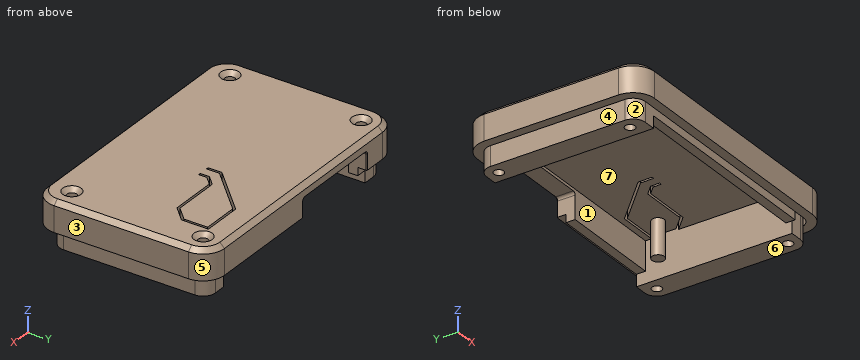
```python
from build123d import *

# Parameters (mm, degrees)
PAD002_DEPTH    = 9.9
POCKET004_DEPTH = 10
PAD003_DEPTH    = 16.4
SKETCH011_W     = 67.75
SKETCH011_H     = 3
PAD004_DEPTH    = 12.5
POCKET005_DEPTH = 13
SKETCH010_R     = 1.6
POCKET006_DEPTH = 19.401
SKETCH012_R     = 2
PAD005_DEPTH    = 14.6
POCKET007_DEPTH = 3
CHAMFER_SIZE    = 1.5
CHAMFER002_SIZE = 1.4
CHAMFER004_SIZE = 0.25


with BuildPart() as part:
    # Sketch006 → Pad002 (new body)
    with BuildSketch(Plane.XY.offset(18)):
        with BuildLine():
            ThreePointArc((-18.5, 103), (-23.449747, 100.949747), (-25.5, 96))
            Line((-25.5, 52), (-25.5, 96))
            ThreePointArc((-25.5, 52), (-23.449747, 47.050253), (-18.5, 45))
            Line((57.25, 45), (-18.5, 45))
            ThreePointArc((57.25, 45), (62.199747, 47.050253), (64.25, 52))
            Line((64.25, 96), (64.25, 52))
            ThreePointArc((64.25, 96), (62.199747, 100.949747), (57.25, 103))
            Line((-18.5, 103), (57.25, 103))
        make_face()
    extrude(amount=-PAD002_DEPTH)

    # Sketch007 → Pocket004 (cut)
    with BuildSketch(Plane.XY.offset(15)):
        with BuildLine():
            ThreePointArc((-18.5, 100), (-21.328427, 98.828427), (-22.5, 96))
            Line((-22.5, 52), (-22.5, 96))
            ThreePointArc((-22.5, 52), (-21.328427, 49.171573), (-18.5, 48))
            Line((57.25, 48), (-18.5, 48))
            ThreePointArc((57.25, 48), (60.078427, 49.171573), (61.25, 52))
            Line((61.25, 96), (61.25, 52))
            ThreePointArc((61.25, 96), (60.078427, 98.828427), (57.25, 100))
            Line((-18.5, 100), (57.25, 100))
        make_face()
    extrude(amount=-POCKET004_DEPTH, mode=Mode.SUBTRACT)

    # Sketch008 → Pad003 (join)
    with BuildSketch(Plane.XY.offset(18)):
        with BuildLine():
            ThreePointArc((-22.5, 52), (-21.328427, 49.171573), (-18.5, 48))
            Line((-14.5, 48), (-18.5, 48))
            Line((-14.5, 100), (-14.5, 48))
            Line((-18.5, 100), (-14.5, 100))
            ThreePointArc((-18.5, 100), (-21.328427, 98.828427), (-22.5, 96))
            Line((-22.5, 52), (-22.5, 96))
        make_face()
        with BuildLine():
            ThreePointArc((61.25, 96), (60.078427, 98.828427), (57.25, 100))
            Line((53.25, 100), (57.25, 100))
            Line((53.25, 49), (53.25, 100))
            Line((57.25, 49), (53.25, 49))
            ThreePointArc((57.25, 49), (60.078427, 50.171573), (61.25, 53))
            Line((61.25, 96), (61.25, 53))
        make_face()
    extrude(amount=-PAD003_DEPTH)

    # Sketch011 → Pad004 (join)
    with BuildSketch(Plane.XY.offset(18)):
        with Locations((19.375, 98.5)):
            Rectangle(SKETCH011_W, SKETCH011_H)
        with Locations((19.375, 49.5)):
            Rectangle(SKETCH011_W, SKETCH011_H)
    extrude(amount=-PAD004_DEPTH)

    # Sketch009 → Pocket005 (cut)
    with BuildSketch(Plane(origin=(0, 108, 0), x_dir=(-1, 0, 0), z_dir=(0, 1, 0))):
        with BuildLine():
            ThreePointArc((-18.65, 14.05), (-19.286396, 13.786396), (-19.55, 13.15))
            Line((-19.55, 2.65), (-19.55, 13.15))
            ThreePointArc((-19.55, 2.65), (-19.286396, 2.013604), (-18.65, 1.75))
            Line((10.15, 1.75), (-18.65, 1.75))
            ThreePointArc((10.15, 1.75), (10.786396, 2.013604), (11.05, 2.65))
            Line((11.05, 13.15), (11.05, 2.65))
            ThreePointArc((11.05, 13.15), (10.786396, 13.786396), (10.15, 14.05))
            Line((-18.65, 14.05), (10.15, 14.05))
        make_face()
    extrude(amount=-POCKET005_DEPTH, mode=Mode.SUBTRACT)

    # Sketch010 → Pocket006 (cut, through all)
    with BuildSketch(Plane.XY.offset(21)):
        with Locations((-18.5, 96)):
            Circle(SKETCH010_R)
        with Locations((-18.5, 53)):
            Circle(SKETCH010_R)
        with Locations((57.25, 53)):
            Circle(SKETCH010_R)
        with Locations((57.25, 96)):
            Circle(SKETCH010_R)
    extrude(amount=-POCKET006_DEPTH, mode=Mode.SUBTRACT)

    # Sketch012 → Pad005 (join)
    with BuildSketch(Plane.XY.offset(18)):
        with Locations((46.5, 88.25)):
            Circle(SKETCH012_R)
    extrude(amount=-PAD005_DEPTH)

    # Sketch013 → Pocket007 (cut)
    with BuildSketch(Plane.XY.offset(18)):
        Polygon((40.5, 94.25), (52.5, 94.25), (52.5, 86.492641), (48.257359, 82.25), (40.5, 82.25), (32.742641, 82.25), (29.742641, 79.25), (29.742641, 76.25), (30.492641, 76.25), (30.492641, 78.93934), (33.053301, 81.5), (48.568019, 81.5), (53.25, 86.181981), (53.25, 95), (40.18934, 95), (25.992641, 80.803301), (25.992641, 76.25), (26.742641, 76.25), (26.742641, 80.492641), align=None)
    extrude(amount=-POCKET007_DEPTH, mode=Mode.SUBTRACT)

    # Chamfer
    chamfer_edges = [part.edges().sort_by_distance(p)[0] for p in [
        (64.25, 74, 18),
    ]]
    chamfer(chamfer_edges, length=CHAMFER_SIZE)

    # Chamfer002
    chamfer002_edges = [part.edges().sort_by_distance(p)[0] for p in [
        (55.65, 96, 18),
        (55.65, 53, 18),
        (-20.1, 53, 18),
        (-20.1, 96, 18),
    ]]
    chamfer(chamfer002_edges, length=CHAMFER002_SIZE)

    # Chamfer004
    chamfer004_edges = [part.edges().sort_by_distance(p)[0] for p in [
        (19.55, 103, 10.625),
    ]]
    chamfer(chamfer004_edges, length=CHAMFER004_SIZE)


solid = part.part
```
Can you work these out from the model? Positions are in its coordinate system, mm. Face numbers are marked on the shaded views. A direction names the side the tool comes from. Round coordinates to 2 decimals unless told otherwise and drop trailing zeros. Order: outer loops, then holes, each group sorted by start corner. A loop starts at its lowest first (then second) coordinate and runs counter-clockwise, first axis right, second up. Notation, with made-up numbers: (35.25, 19) -> (57.25, 19) arc R31 cw to (57.25, 46) -> close; hole circle Ø2 at (22, 35.5). An arc over 180 degrees is marked (long way). Return JSON: item names as keys, results as strings. Group by question number.
1. If we section it at B-B, the plane x = 46.5: Write out the boundary of the cut face in (y, z).
2. If we section it at A-A, the plane z = 11: Count the separate pieces of the cut face and the enclosed holes in it, then the cut area to 3 significant figures.
3. If we section it at C-C, the plane y = 72.5: Write out the boundary of the cut face in (x, z).
4. I need wall thicknesses on line 1 (X direction, y = 96, z = 8.5); line 2 (Y direction, x = -18.5, z = 7.25); line 3 (Y direction, x = 57.5, z = 15.75). Which ranges of each line are inside material? Lowest first, please. Write a range as [from, to].
5. If we section it at D-D, the plane x = 15: Write out the boundary of the cut face in (y, z), then the cut area to 3 significant figures.
6. Which directions (+Z, -Z, +X, -X, +Y, -Y) give clear straight access to the entire face, cutting with the end or side of a thin tool? Please do the marked faces 1, 2 and 3.
7. Will these pins go through, and if not, where does the flat tip stop? pin 1 (0.9 mm diameter, centred on x = 28, y = 99, fed in from -Z); pin 2 (1.9 mm diameter, centred on x = 14.5, z = 6, fed in from -Y); pin 3 (7.5 mm diameter, centred on x = 8, z = 9.5, fed in from +Y).
8. We'd pull the mould along X, two halves only. Please class the marked faces 4, 5, 6 and 7: released by +X, released by -X, zero draft, split by the parting line, or undercut.
Output values:
{
 "1": {"outline": "(45, 8.1) -> (48, 8.1) -> (48, 5.5) -> (51, 5.5) -> (51, 15) -> (81.5, 15) -> (81.5, 18) -> (46.5, 18) -> (45, 16.5) -> close; (82.25, 15) -> (86.25, 15) -> (86.25, 3.4) -> (90.25, 3.4) -> (90.25, 15) -> (94.25, 15) -> (94.25, 18) -> (82.25, 18) -> close; (95, 15) -> (97, 15) -> (97, 5.5) -> (100, 5.5) -> (100, 8.1) -> (103, 8.1) -> (103, 16.5) -> (101.5, 18) -> (95, 18) -> close"},
 "2": {"separate pieces": "2", "enclosed holes": "5", "area": "1,840 mm²"},
 "3": {"outline": "(-25.5, 8.1) -> (-22.5, 8.1) -> (-22.5, 1.6) -> (-14.5, 1.6) -> (-14.5, 15) -> (53.25, 15) -> (53.25, 1.6) -> (61.25, 1.6) -> (61.25, 8.1) -> (64.25, 8.1) -> (64.25, 16.5) -> (62.75, 18) -> (-24, 18) -> (-25.5, 16.5) -> close"},
 "4": {"line 1": "[-25.5, -20.1], [-16.9, -14.5], [53.25, 55.65], [58.85, 64.25]", "line 2": "[48, 51.4], [54.6, 94.4], [97.6, 100]", "line 3": "[45, 51.42], [54.58, 94.42], [97.58, 103]"},
 "5": {"outline": "(45, 8.1) -> (48, 8.1) -> (48, 5.5) -> (51, 5.5) -> (51, 15) -> (97, 15) -> (97, 14.05) -> (102.75, 14.05) -> (103, 14.3) -> (103, 16.5) -> (101.5, 18) -> (46.5, 18) -> (45, 16.5) -> close", "area": "227 mm²"},
 "6": {"face 1": "-Z", "face 2": "-Z, -X, -Y", "face 3": "+Z, -Z, +X, +Y, -Y"},
 "7": {"pin 1": "z = 5.5", "pin 2": "y = 48", "pin 3": "y = 51"},
 "8": {"face 4": "released by -X", "face 5": "released by +X", "face 6": "zero draft", "face 7": "undercut"}
}
